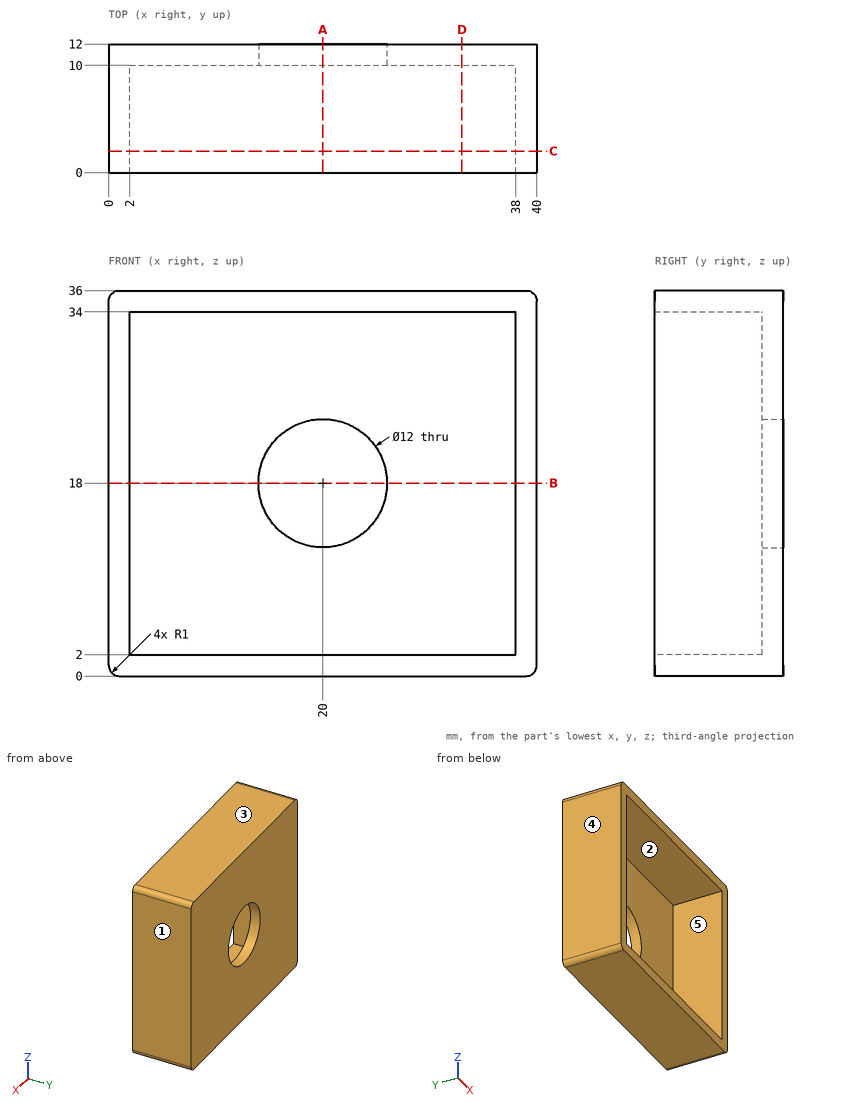
Input: dimensioned drawing with shaded views. Units: mm. Origin: part minimum x, y, z. A direction names the side the tool comes from. Coordinates: 2 decimals unless noted, no trailing zeros. Order: outer loops, then holes, each group sorted by start corner. A loop starts at its lowest first (then second) coordinate and runs counter-clockwise, first axis right, second up. Notation, with made-up numbers: (85, 32) -> (100, 32) arc R22 cw to (100, 45) -> close; hole circle Ø11 at (-25.75, -18). An arc over 180 degrees is marked (long way). Answer in a Markdown table with one row per item.
Item 1: Ray query, L1, parallel to X at y = 3.25, z = 19; L2, parallel to Z at x = 24.5, y = 8; L3, parallel to Z at x = 20, y = 10.6. Return the intervals inside material, ascending.
Return value:
| item | result |
|---|---|
| L1 | x = 0 to 2, 38 to 40 |
| L2 | z = 0 to 2, 34 to 36 |
| L3 | z = 0 to 12, 24 to 36 |
Item 2: Section C-C on y = 2. Output: boundary loops of the cut face in (x, z).
Return value:
| item | result |
|---|---|
| outline | (0, 1) arc R1 ccw to (1, 0) -> (39, 0) arc R1 ccw to (40, 1) -> (40, 35) arc R1 ccw to (39, 36) -> (1, 36) arc R1 ccw to (0, 35) -> close; hole (2, 2) -> (38, 2) -> (38, 34) -> (2, 34) -> close |
Item 3: Draft query along Z for the marked faces 3, 4 and 5. Return one class per face: released by +Z, released by -Z, zero draft, split by the parting line, or undercut.
Return value:
| item | result |
|---|---|
| face 3 | released by +Z |
| face 4 | zero draft |
| face 5 | undercut |
Item 4: Contact query for a flat-ended pin moving along its axis: P1, Ø9.5, axis at x = 25, z = 26, coming from the -Y side. Output: stop coordinate, or through.
Return value:
| item | result |
|---|---|
| P1 | stops at y = 10 |
Item 5: Section A-A on x = 20. Output: boundary loops of the cut face in (y, z), plus the area to 3 significant figures.
Return value:
| item | result |
|---|---|
| outline | (0, 0) -> (12, 0) -> (12, 12) -> (10, 12) -> (10, 2) -> (0, 2) -> close; (0, 34) -> (10, 34) -> (10, 24) -> (12, 24) -> (12, 36) -> (0, 36) -> close |
| area | 88.0 mm² |
Item 6: Section B-B on z = 18. Output: boundary loops of the cut face in (x, y).
Return value:
| item | result |
|---|---|
| outline | (0, 0) -> (2, 0) -> (2, 10) -> (14, 10) -> (14, 12) -> (0, 12) -> close; (26, 10) -> (38, 10) -> (38, 0) -> (40, 0) -> (40, 12) -> (26, 12) -> close |
Item 7: Section D-D on x = 33. Output: boundary loops of the cut face in (y, z).
Return value:
| item | result |
|---|---|
| outline | (0, 0) -> (12, 0) -> (12, 36) -> (0, 36) -> (0, 34) -> (10, 34) -> (10, 2) -> (0, 2) -> close |
Item 8: Access query for the marked faces 1 and 2. Directions: +Z, -Z, +X, -X, +Y, -Y. A direction counts if a zero-diameter tool reaches every point of the face in a straight line with its end or side. Return the directions, or none.
Return value:
| item | result |
|---|---|
| face 1 | +Z, -Z, +X, +Y, -Y |
| face 2 | -Y |
